For this review, take the finished solid that the model builds, in its own axes (mm). A direction names the side the tool comes from. Give positions to 0.01 mm unless a question says otherwise; leave off trailing zeros. Order: outer loops, then holes, each group sorted by start corner. A loop starts at its lowest first (then second) coordinate and runs counter-clockwise, first axis right, second up.
Item 1: For probe 1 along Y at (x, z) = (35, 18); probe 2 along Z at (x, y) = (5.5, 1.5); probe 3 along Y at (x, z) = (31, 2), list the stretches that pass through material, from the lowest coordinate up.
Item 2: The part is to be moulded in two halves that separate along Y. For faces 1 (the flat face through (19, 25.4, 16)), 2 (the flat face through (13, 0, 6)), 3 (the flat face through (19, 19, 31.75)), say which applies: released by +Y, released by -Y, zero draft, split by the parting line, or undercut.
Item 3: For P1, Ø2, axis at x = 14, z = 24, coming from the -Y side; P2, Ø6.5, axis at x = 20, y = 4, coming from the +Z side, all flat-tipped, find the tip position at first contact; note any pin that passes through.
Item 4: Consider section C-C (y = 7). Give the boundary of the cut face in (x, z).
Item 5: Machinability: for faces 4 (the flat face through (19, 13, 0)), 5 (the flat face through (15, 6, 12.7)), which of the approach directions +Z, -Z, +X, -X, +Y, -Y give a long, thin tool a straight path to every point of the face, cutting with its end or side? Answer none if there is none.
Item 6: Consider section D-D (x = 31). Give the boundary of the cut face in (y, z).
Item 7: Consider section B-B (x = 4). Give the boundary of the cut face in (y, z).
Item 8: Consider section A-A (z = 9). Give the boundary of the cut face in (x, y).
```python
from build123d import *

# Parameters (mm, degrees)
F1_DEPTH = 38.1
F3_DEPTH = 25.4


with BuildPart() as f1:
    # F0 (on Right) → F1 (new body)
    with BuildSketch(Plane.YZ):
        Polygon((0, 12.7), (0, 0), (25.4, 0), (25.4, 31.75), (12.7, 31.75), (12.7, 12.7), align=None)
    extrude(amount=F1_DEPTH)

    # F2 (on Top) → F3 (cut)
    with BuildSketch(Plane.XY):
        Polygon((26.027159, 0), (38.727159, 0), (38.727159, 12.7), align=None)
    extrude(amount=F3_DEPTH, mode=Mode.SUBTRACT)


solid = f1.part
```
Resolved:
1. probe 1: y = 12.7 to 25.4
1. probe 2: z = 0 to 12.7
1. probe 3: y = 4.97 to 25.4
2. face 1: released by +Y
2. face 2: released by -Y
2. face 3: zero draft
3. P1: stops at y = 12.7
3. P2: stops at z = 12.7
4. outline: (0, 0) - (33.03, 0) - (33.03, 12.7) - (0, 12.7) - close
5. face 4: -Z, +X, -X, +Y, -Y
5. face 5: +Z, +X, -X, -Y
6. outline: (4.97, 0) - (25.4, 0) - (25.4, 31.75) - (12.7, 31.75) - (12.7, 12.7) - (4.97, 12.7) - close
7. outline: (0, 0) - (25.4, 0) - (25.4, 31.75) - (12.7, 31.75) - (12.7, 12.7) - (0, 12.7) - close
8. outline: (0, 0) - (26.03, 0) - (38.1, 12.07) - (38.1, 25.4) - (0, 25.4) - close
